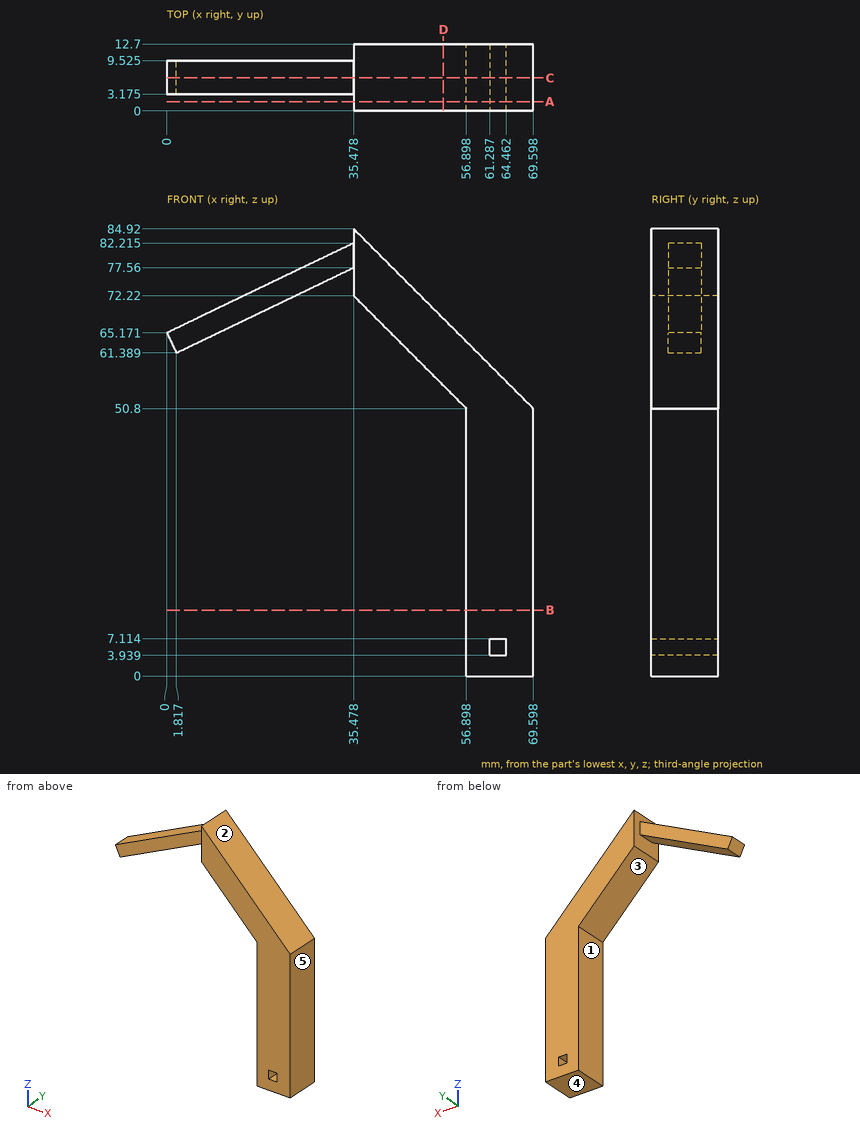
The figure shows three views and two pictorial views of one solid part (mm, origin at its lowest corner). Answer the questions. A direction names the side the tool comes from. Give positions to 0.01 mm unless a question says otherwise; leave off trailing zeros. Loops run counter-clockwise (first coordinate to the right, second up) from the corner with the lowest first, then second, coordinate; pieces in that order, holes last. Notation, with made-up numbers: (53.25, 71) - (103.25, 71) arc R12 cw to (103.25, 83) - close; hole circle Ø4 at (-26.5, 37.5). An arc over 180 degrees is marked (long way). Answer in a Markdown table with one row per item.
(1) Consider L1, parallel to X at y = 9, z = 46; L2, parallel to Y at x = 34, z = 80.5 (1 decimal); L3, parallel to Z at x = 62.5, y = 5 (1 decimal). Determine where each line is inside the solid, lowest interval first. Write a range as [from, to].
Results list:
| item | result |
|---|---|
| L1 | x = [56.9, 69.6] |
| L2 | y = [3.2, 9.5] |
| L3 | z = [0, 3.9], [7.1, 57.9] |
(2) A tool of negligible diameter and unlimited length cuts with its end or side. For the marked faces 1 and 2, from which of +Z, -Z, +X, -X, +Y, -Y can it reach the whole face along a straight path? Write none if from no direction.
Results list:
| item | result |
|---|---|
| face 1 | -Z, -X, +Y, -Y |
| face 2 | +Z, +X, +Y, -Y |
(3) Section A-A (y = 1.75) is taken. Give the vertices of the cut face in (x, z), and give its area (3 significant figures).
Results list:
| item | result |
|---|---|
| outline | (35.48, 72.22) - (56.9, 50.8) - (56.9, 0) - (69.6, 0) - (69.6, 50.8) - (35.48, 84.92) - close; hole (61.29, 3.94) - (64.46, 3.94) - (64.46, 7.11) - (61.29, 7.11) - close |
| area | 988 mm² |
(4) Flat-ended cylindrical pins translate along their axes: pin 1 Ø3 at (x, y) = (52, 6.5) entering from -Z; pin 2 Ø16.5 at (x, z) = (26, 67) entering from -Y (3 decimals); pin 3 Ø10.5 at (x, z) = (21, 69.5) entering from +Y (3 decimals); pin 4 Ø1 at (x, y) = (62.5, 8.5) entering from -Z. Find the tip coordinate at first contact, or state that the pin passes through.
Results list:
| item | result |
|---|---|
| pin 1 | stops at z = 54.2 |
| pin 2 | stops at y = 3.175 |
| pin 3 | stops at y = 9.525 |
| pin 4 | stops at z = 0 |
(5) For a pull along X with two mould halves and no side action, classify the marked faces 3, 4 and 5 as pulls with the +X half, pulls with the -X half, needs draft (parallel to the pull), parting line crosses it, or undercut.
Results list:
| item | result |
|---|---|
| face 3 | undercut |
| face 4 | needs draft |
| face 5 | pulls with the +X half |
(6) Section D-D (x = 52.5) is taken. Give the vertices of the cut face in (y, z), and give its area (3 significant figures).
Results list:
| item | result |
|---|---|
| outline | (0, 55.2) - (12.7, 55.2) - (12.7, 67.9) - (0, 67.9) - close |
| area | 161 mm² |
(7) Section C-C (y = 6.25) is taken. Give the vertices of the cut face in (x, z) (1 decimal), and give its area (3 significant figures).
Results list:
| item | result |
|---|---|
| outline | (0, 65.2) - (1.8, 61.4) - (35.5, 77.6) - (35.5, 72.2) - (56.9, 50.8) - (56.9, 0) - (69.6, 0) - (69.6, 50.8) - (35.5, 84.9) - (35.5, 82.2) - close; hole (61.3, 3.9) - (64.5, 3.9) - (64.5, 7.1) - (61.3, 7.1) - close |
| area | 1,150 mm² |
(8) Section B-B (z = 12.5) is taken. Give the vertices of the cut face in (x, y).
Results list:
| item | result |
|---|---|
| outline | (56.9, 0) - (69.6, 0) - (69.6, 12.7) - (56.9, 12.7) - close |
